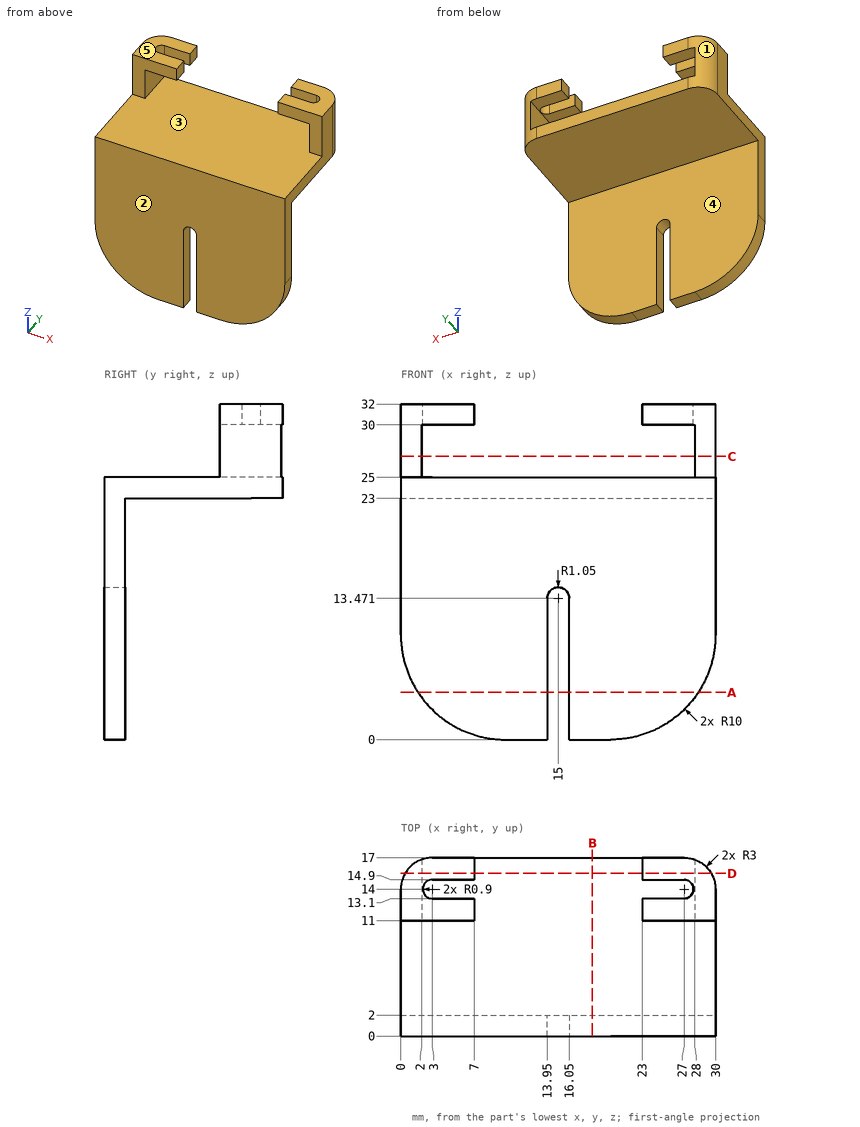
For this review, use the dimensioned drawing (mm, ordinates from the lowest corner) and the shaded views. A direction names the side the tool comes from. Round coordinates to 2 decimals unless told otherwise and drop trailing zeros. Write each loop counter-clockwise with the first axis right and the second up, starting at its lowest first coordinate (ties: lowest second). Pieces come first, ordered by that corner, then holes. Notation, with made-up numbers: (23, -35) -> (65, -35) arc R24 ccw to (65, -16) -> close; hole circle Ø5 at (-38.5, 50). An arc over 180 degrees is marked (long way). Answer in a Markdown table with one row per item.
Q1. To check wall thickness, follow L1, parallel to Z at x = 6.75, y = 13; L2, parallel to Y at x = 18.25, z = 3; L3, parallel to Z at x = 7.25, y = 12. State the ranges of each line that lie inside material, in increasing order. Write a range as [from, to].
The answers:
| item | result |
|---|---|
| L1 | [23, 25], [30, 32] |
| L2 | [0, 2] |
| L3 | [23, 25] |
Q2. Take a section at A-A, the plane z = 4.5. State the section outline as (x, y) points, then the cut area to 3 significant figures.
The answers:
| item | result |
|---|---|
| outline | (1.65, 0) -> (13.95, 0) -> (13.95, 2) -> (1.65, 2) -> close; (16.05, 0) -> (28.35, 0) -> (28.35, 2) -> (16.05, 2) -> close |
| area | 49.2 mm² |
Q3. Take a section at D-D, the plane y = 15.5. State the section outline as (x, z) points, then the cut area to 3 significant figures.
The answers:
| item | result |
|---|---|
| outline | (0.4, 23) -> (29.6, 23) -> (29.6, 32) -> (23, 32) -> (23, 30) -> (28, 30) -> (28, 25) -> (2, 25) -> (2, 30) -> (7, 30) -> (7, 32) -> (0.4, 32) -> close |
| area | 101 mm² |
Q4. Take a section at B-B, the plane x = 18.25. State the section outline as (y, z) points.
The answers:
| item | result |
|---|---|
| outline | (0, 0) -> (2, 0) -> (2, 23) -> (17, 23) -> (17, 25) -> (0, 25) -> close |
Q5. Take a section at C-C, the plane z = 27. State the section outline as (x, y) points.
The answers:
| item | result |
|---|---|
| outline | (0, 11) -> (2, 11) -> (2, 16.83) arc R3 ccw to (0, 14) -> close; (28, 11) -> (30, 11) -> (30, 14) arc R3 ccw to (28, 16.83) -> close |
Q6. For the marked faces 4 and 5, list the 3-axis set-ups (+Z, -Z, +X, -X, +Y, -Y) from which the entire face can be reached by the end or side of a thin tool; tool diameter is ignored.
The answers:
| item | result |
|---|---|
| face 4 | -Z, +X, -X, +Y |
| face 5 | +Z, +X, -X, +Y, -Y |
Q7. Draft analysis for pull direction Y (two halves, no side actions). For the marked faces 1, 2 and 3, state which applies: +Y half, -Y half, draft (parallel to the pull), parting line (faces both ways), or undercut.
The answers:
| item | result |
|---|---|
| face 1 | +Y half |
| face 2 | -Y half |
| face 3 | draft |
Q8. Clearance check with flat-ended pins moving along their axes: pin 1 Ø11.5 at (x, z) = (10.5, 10.5) entering from +Y; pin 2 Ø2 at (y, z) = (1, 4) entering from -X; pin 3 Ø5 at (x, y) = (13, 11) entering from +Z. State where each tip first meets the part, or that it passes through.
The answers:
| item | result |
|---|---|
| pin 1 | y = 2 |
| pin 2 | x = 1.34 |
| pin 3 | z = 25 |
